Can you work these out from the model? Positions are in its coordinate system, mm. A direction names the side the tool comes from. Coordinates: 2 decimals unless noted, no trailing zeros. Loops run counter-clockwise (first coordinate to the right, second up) from the corner with the lowest first, then second, coordinate; pieces in that order, holes last. Notation, with made-up numbers: (19, -35) -> (61, -35) arc R20 ccw to (61, -6) -> close; hole circle Ø10 at (14, 66.5). An arc over 180 degrees is marked (long way). Put each result on its own line as item: value. Start each with the question number.
Item 1: We'd pull the mould along Y, two halves only. Please class faces 1 (the flat face through (40, 5, 0)), 2 (the flat face through (-15, 12.5, 0)), 3 (the flat face through (-29.302, 19.86, 0.14)): pulls with the +Y half, pulls with the -Y half, needs draft (parallel to the pull), parting line crosses it, or undercut.
Item 2: If we section it at D-D on x = 2: Please give me the cut outline in (y, z).
Item 3: If we section it at A-A on y = 7: Please give me the cut outline in (x, z).
Item 4: If we section it at C-C on y = 24: Please give me the cut outline in (x, z).
Item 5: Will these pins go through, and if not, where does the flat tip stop? P1, Ø6, axis at x = -30, y = 20.5, coming from the -Z side; P2, Ø0.9, axis at y = 48, z = 7, coming from the +X side; P3, Ø11, axis at x = -18, y = 33, coming from the +Z side; P4, Ø4, axis at x = -33, z = 33, coming from the -Y side.
Item 6: If we section it at B-B on z = 13.5: Please give me the cut outline in (x, y), plus the area to 3 significant figures.
Item 7: Please list where these lines run through material, in increasing order: L1, parallel to Z at x = -14.5, y = 14.35; L2, parallel to X at y = 6, z = 33. Write a range as from..to.
Item 8: For faces 4 (the flat face through (-15, 49, 9)), 5 (the flat face through (-11.5, 49, 0)), 6 (the flat face through (-22, 30, -16)), 7 (the flat face through (-25.5, 34, 0)), which set-ups out of +Z, -Z, +X, -X, +Y, -Y let a thin tool reach every point of the face, with its end or its side?
```python
from build123d import *

# Parameters (mm, degrees)
SKETCH1_R           = 2.5
BOSS_EXTRUDE1_DEPTH = 10
SKETCH5_W           = 8
SKETCH5_H           = 32
BOSS_EXTRUDE4_DEPTH = 40
BOSS_EXTRUDE5_DEPTH = 10
SKETCH7_W           = 32
SKETCH7_H           = 3
BOSS_EXTRUDE6_DEPTH = 6
SKETCH8_R           = 0.5
CUT_EXTRUDE1_DEPTH  = 39
SKETCH9_R           = 1.5
CUT_EXTRUDE2_DEPTH  = 1


with BuildPart() as part:
    # Sketch1 → Boss-Extrude1 (new body)
    with BuildSketch(Plane(origin=(0, 0, 0), x_dir=(1, 0, 0), z_dir=(0, 1, 0))):
        with BuildLine():
            Line((-33, -40), (33, -40))
            ThreePointArc((33, -40), (37.949747468, -37.949747468), (40, -33))
            Line((40, -33), (40, 33))
            ThreePointArc((40, 33), (37.949747468, 37.949747468), (33, 40))
            Line((33, 40), (-33, 40))
            ThreePointArc((-33, 40), (-37.949747468, 37.949747468), (-40, 33))
            Line((-40, 33), (-40, -33))
            ThreePointArc((-40, -33), (-37.949747468, -37.949747468), (-33, -40))
        make_face()
        with Locations((33, -33)):
            Circle(SKETCH1_R, mode=Mode.SUBTRACT)
        with Locations((-33, -33)):
            Circle(SKETCH1_R, mode=Mode.SUBTRACT)
        with Locations((33, 33)):
            Circle(SKETCH1_R, mode=Mode.SUBTRACT)
        with Locations((-33, 33)):
            Circle(SKETCH1_R, mode=Mode.SUBTRACT)
    extrude(amount=BOSS_EXTRUDE1_DEPTH)

    # Sketch5 → Boss-Extrude4 (add)
    with BuildSketch(Plane(origin=(0, 10, 0), x_dir=(1, 0, 0), z_dir=(0, 1, 0))):
        with Locations((-21.5, 0)):
            Rectangle(SKETCH5_W, SKETCH5_H)
    extrude(amount=BOSS_EXTRUDE4_DEPTH)

    # Sketch6 → Boss-Extrude5 (add, symmetric)
    with BuildSketch(Plane.XY):
        Polygon((-33, 10), (-25.5, 30), (-25.5, 10), align=None)
    extrude(amount=BOSS_EXTRUDE5_DEPTH, both=True)

    # Sketch7 → Boss-Extrude6 (add)
    with BuildSketch(Plane(origin=(-17.5, 0, 0), x_dir=(0, 0, -1), z_dir=(1, 0, 0))):
        with Locations((0, 48.5)):
            Rectangle(SKETCH7_W, SKETCH7_H)
        with Locations((0, 14)):
            Rectangle(SKETCH7_W, SKETCH7_H)
    extrude(amount=BOSS_EXTRUDE6_DEPTH)

    # Sketch8 → Cut-Extrude1 (cut)
    with BuildSketch(Plane(origin=(0, 50, 0), x_dir=(1, 0, 0), z_dir=(0, 1, 0))):
        with Locations((-14.5, -8)):
            Circle(SKETCH8_R)
        with Locations((-14.5, 8)):
            Circle(SKETCH8_R)
    extrude(amount=-CUT_EXTRUDE1_DEPTH, mode=Mode.SUBTRACT)

    # Sketch9 → Cut-Extrude2 (cut)
    with BuildSketch(Plane(origin=(0, 50, 0), x_dir=(1, 0, 0), z_dir=(0, 1, 0))):
        with Locations((-14.5, 8)):
            Circle(SKETCH9_R)
        with Locations((-14.5, -8)):
            Circle(SKETCH9_R)
    extrude(amount=-CUT_EXTRUDE2_DEPTH, mode=Mode.SUBTRACT)


solid = part.part
```
Solutions:
1. face 1: needs draft
1. face 2: undercut
1. face 3: pulls with the +Y half
2. outline: (0, -40) -> (10, -40) -> (10, 40) -> (0, 40) -> close
3. outline: (-40, -33) arc R7 ccw to (-33, -40) -> (33, -40) arc R7 ccw to (40, -33) -> (40, 33) arc R7 ccw to (33, 40) -> (-33, 40) arc R7 ccw to (-40, 33) -> close; hole circle Ø5 at (-33, -33); hole circle Ø5 at (-33, 33); hole circle Ø5 at (33, -33); hole circle Ø5 at (33, 33)
4. outline: (-27.75, -10) -> (-25.5, -10) -> (-25.5, -16) -> (-17.5, -16) -> (-17.5, 16) -> (-25.5, 16) -> (-25.5, 10) -> (-27.75, 10) -> close
5. P1: z = -10
5. P2: x = -11.5
5. P3: z = 16
5. P4: through
6. outline: (-40, 0) -> (40, 0) -> (40, 10) -> (-17.5, 10) -> (-17.5, 12.5) -> (-11.5, 12.5) -> (-11.5, 15.5) -> (-17.5, 15.5) -> (-17.5, 47) -> (-11.5, 47) -> (-11.5, 50) -> (-25.5, 50) -> (-25.5, 10) -> (-40, 10) -> close
6. area: 1,160 mm^2
7. L1: -16..-8.5, -7.5..7.5, 8.5..16
7. L2: -40..-35.5, -30.5..30.5, 35.5..40
8. face 4: +Y
8. face 5: +Z, -Z, +X, +Y
8. face 6: -Z, +X, -X, +Y
8. face 7: -X, +Y
